Input: dimensioned drawing with shaded views. Units: mm. Origin: part minimum x, y, z. Round coordinates to 2 decimals unless told otherwise and drop trailing zeros. Write each loop counter-clockwise with the first axis right and the second up, starting at its lowest first coordinate (ties: lowest second). Pieces come first, ordered by that corner, then holes. Notation, with made-up numbers: (34, 43.5) - (58, 43.5) arc R23 ccw to (58, 55.5) - close; hole circle Ø9 at (27, 36.25). An arc over 180 degrees is marked (long way). Write item = value, one per line. Start each with the question number.
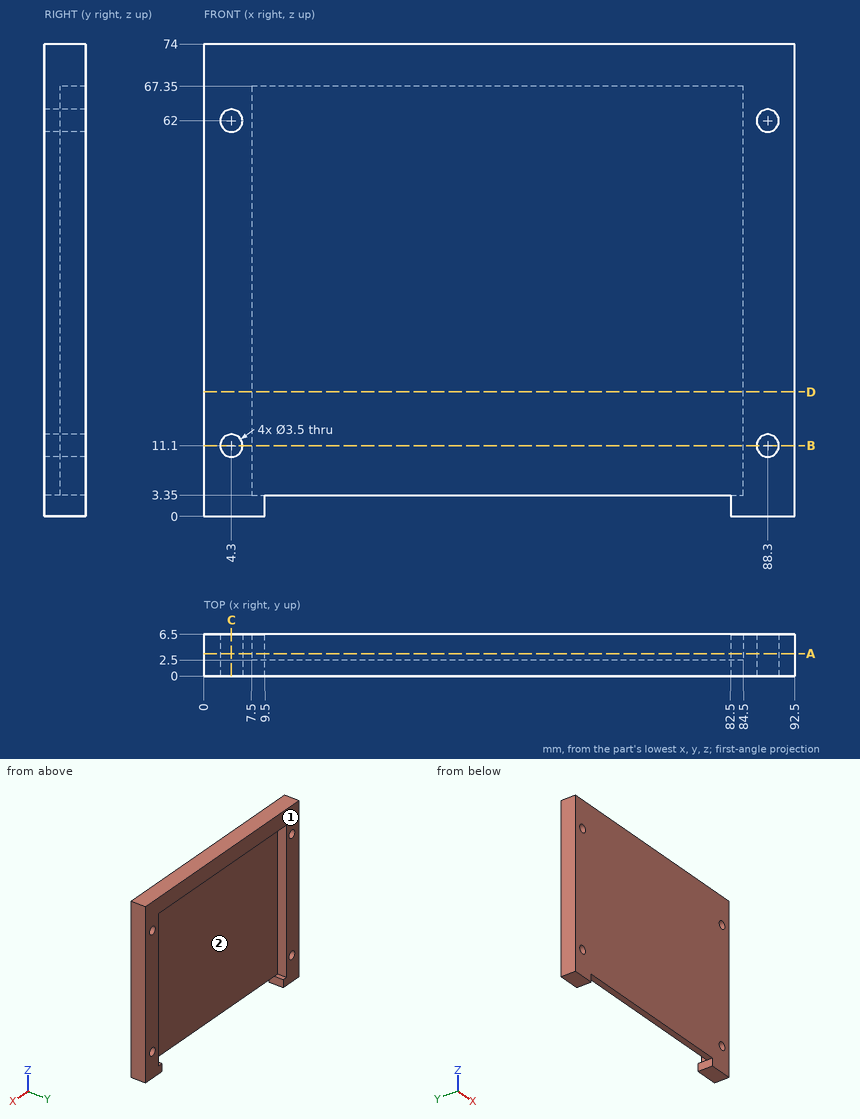
(1) Pull-direction query (X, two-part tool) for the marked faces 1 and 2; classes: +X half, -X half, draft (parallel to the pull), parting line (faces both ways), or undercut.
(2) Section B-B (z = 11.1). Return the cut outline in (x, y), plus the area to 3 significant figures.
(3) Contact query for flat-ended pins moving along their axis: P1, Ø3, axis at x = 4.3, z = 62, coming from the -Y side; P2, Ø2, axis at x = 63, y = 4.5, coming from the -Z side; P3, Ø1.2, axis at x = 43, y = 1, coming from the -Z side. Output: stop coordinate, or through.
(4) Section C-C (x = 4.3). Return the cut outline in (y, z).
(5) Section D-D (z = 19.5). Return the cut outline in (x, y), plus the area to 3 significant figures.
(6) Ray query, L1, parallel to Z at x = 4.3, y = 3.5; L2, parallel to Z at x = 84, y = 4.5; L3, parallel to X at y = 4, z = 62. Return the intervals inside material, ascending. Write a range as from..to.
(7) Section A-A (y = 3.5). Return the cut outline in (x, z), plus the area to 3 significant figures.
Solution:
q1.face_1 = draft
q1.face_2 = undercut
q2.outline = (0, 0) - (2.55, 0) - (2.55, 6.5) - (0, 6.5) - close; (6.05, 0) - (86.55, 0) - (86.55, 6.5) - (84.5, 6.5) - (84.5, 2.5) - (7.5, 2.5) - (7.5, 6.5) - (6.05, 6.5) - close; (90.05, 0) - (92.5, 0) - (92.5, 6.5) - (90.05, 6.5) - close
q2.area = 248 mm^2
q3.P1 = through
q3.P2 = 67.35
q3.P3 = 3.35
q4.outline = (0, 0) - (6.5, 0) - (6.5, 9.35) - (0, 9.35) - close; (0, 12.85) - (6.5, 12.85) - (6.5, 60.25) - (0, 60.25) - close; (0, 63.75) - (6.5, 63.75) - (6.5, 74) - (0, 74) - close
q5.outline = (0, 0) - (92.5, 0) - (92.5, 6.5) - (84.5, 6.5) - (84.5, 2.5) - (7.5, 2.5) - (7.5, 6.5) - (0, 6.5) - close
q5.area = 293 mm^2
q6.L1 = 0..9.35, 12.85..60.25, 63.75..74
q6.L2 = 0..3.35, 67.35..74
q6.L3 = 0..2.55, 6.05..7.5, 84.5..86.55, 90.05..92.5
q7.outline = (0, 0) - (9.5, 0) - (9.5, 3.35) - (7.5, 3.35) - (7.5, 67.35) - (84.5, 67.35) - (84.5, 3.35) - (82.5, 3.35) - (82.5, 0) - (92.5, 0) - (92.5, 74) - (0, 74) - close; hole circle Ø3.5 at (4.3, 11.1); hole circle Ø3.5 at (4.3, 62); hole circle Ø3.5 at (88.3, 11.1); hole circle Ø3.5 at (88.3, 62)
q7.area = 1,630 mm^2
